```python
from build123d import *

# Parameters (mm, degrees)
SKETCH024_W                = 7
SKETCH024_H                = 2
SKETCH024_W_2              = 8
SKETCH024_H_2              = 4
EXTRUDE020_DEPTH           = 5
EXTRUDE020_DEPTH_BACK      = 14
EXTRUDE014_DEPTH           = 27
EXTRUDE014_PLACEMENT_ANGLE = 15


with BuildPart() as extrude020:
    # Sketch024 → Extrude020 (new body, two sides)
    with BuildSketch(Plane.XZ) as extrude020_sk:
        with Locations((13.5, 19)):
            Rectangle(SKETCH024_W, SKETCH024_H)
        with Locations((20, 45)):
            Rectangle(SKETCH024_W_2, SKETCH024_H_2)
    extrude(amount=EXTRUDE020_DEPTH)
    extrude(extrude020_sk.sketch, amount=-EXTRUDE020_DEPTH_BACK)


with BuildPart() as cut001:
    # Sketch018 → Extrude014 (new body)
    with BuildSketch(Plane.XY.offset(45)):
        Polygon((20, 9), (22, 9), (22, 11), (18, 11), (18, -2), (22, -2), (22, 0), (20, 0), align=None)
    extrude(amount=-EXTRUDE014_DEPTH)


with BuildPart() as cut001_1:
    # Extrude014 placement: moved
    add(cut001.part.moved(Location((-11, 0, 7))).rotate(Axis((-11, 0, 7), (0, 1, 0)), EXTRUDE014_PLACEMENT_ANGLE))

    # Cut001: cut Extrude020
    add(extrude020.part, mode=Mode.SUBTRACT)


solid = cut001_1.part
```
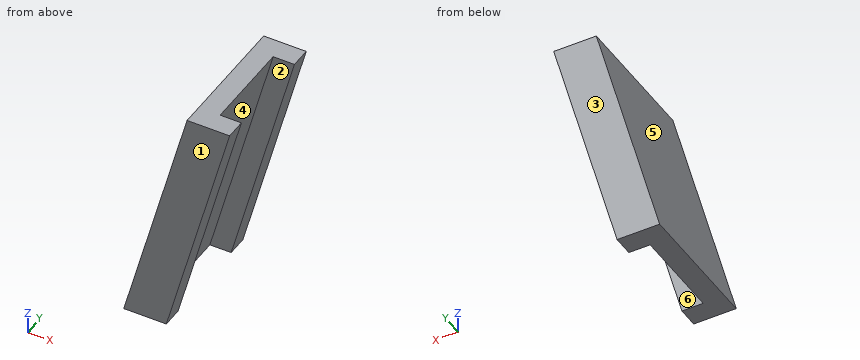
Geometry check sheet. Reference: the model listing, model coordinates, mm. Face numbers are marked on the shaded views. A direction names the side the tool comes from. Round coordinates to 2 decimals unless told otherwise and drop trailing zeros. Loops run counter-clockwise (first coordinate to the right, second up) from the corner with the lowest first, then second, coordinate; pieces in that order, holes last. Notation, with made-up numbers: (51.5, 29) - (56.5, 29) arc R9 cw to (56.5, 38) - close; hole circle Ø4 at (32.25, -21.5). An arc over 180 degrees is marked (long way). Write item = value, one per line. Start each with the question number.
1. Thickness scan on line 1 (Y direction, x = 16.75, z = 30.75); line 2 (X direction, y = 5.5, z = 27.75); line 3 (X direction, y = 5.75, z = 41.25). Record the ranges inside material, lowest first.
2. Set-up check for the marked faces 5 and 6: record each of +Z, -Z, +X, -X, +Y, -Y from which the full face is reachable in a straight line by a thin tool's end or side.
3. Section check C-C on z = 40.75. Enter the section's corners in (x, y).
4. Mould release check, pull along Y, two halves, no side actions. Record for the marked faces 1, 2, 3 and 4: released by +Y, released by -Y, zero draft, split by the parting line, or undercut.
5. Section check A-A on x = 20.5. Enter the section's corners in (y, z), then the cut area to 3 significant figures.
6. Section check D-D on y = 9.25. Enter the section's corners in (x, z).
7. Section check B-B on x = 18.5. Enter the section's corners in (y, z), then the cut area to 3 significant figures.
Working result:
q1.line_1 = -2 to 0, 9 to 11
q1.line_2 = 13.19 to 15.27
q1.line_3 = 16.81 to 18.88
q2.face_5 = +Z, -X, +Y, -Y
q2.face_6 = -Z, +X
q3.outline = (16.68, -2) - (20.82, -2) - (20.82, 0) - (18.75, 0) - (18.75, 9) - (20.82, 9) - (20.82, 11) - (16.68, 11) - close
q4.face_1 = released by -Y
q4.face_2 = undercut
q4.face_3 = released by +Y
q4.face_4 = undercut
q5.outline = (-2, 39.56) - (0, 39.56) - (0, 43) - (-2, 43) - close; (9, 39.56) - (11, 39.56) - (11, 43) - (9, 43) - close
q5.area = 13.8 mm^2
q6.outline = (11.12, 20) - (15.26, 20) - (21.42, 43) - (17.28, 43) - close
q7.outline = (-2, 32.09) - (0, 32.09) - (0, 39.82) - (9, 39.82) - (9, 32.09) - (11, 32.09) - (11, 43) - (-2, 43) - close
q7.area = 72.2 mm^2
